Source: CAD feature listing. Evaluate the final solid. Frame: model axes, mm. Face numbers are marked on the shaded views. A direction names the side the tool comes from. Coordinates: 2 decimals unless noted, no trailing zeros. Write each loop counter-clockwise with the first axis right and the second up, starting at its lowest first coordinate (ties: lowest second). Pieces come first, ordered by that corner, then holes. Notation, with made-up numbers: M 51.5,-10.5 L 100.5,-10.5 A22 cw 100.5,17.5 Z; hole C -1,-37.5 d3. An arc over 180 degrees is marked long. Answer as CSV lines item,"result". Start each with the question number.
1. Line query: probe 1 along X at (y, z) = (211.5, 20.5); probe 2 along X at (y, z) = (152.5, -3); probe 3 along X at (y, z) = (285, -16). Output: solid intervals per line, ascending. Write a range as [from, to].
2. Mould query, pull axis X, two halves, no side actions, for the marked faces 3, 4, 5 and 6. Classes: pulls with the +X half, pulls with the -X half, needs draft (parallel to the pull), parting line crosses it, or undercut.
3. Section B-B on y = 429.5. Return the cut outline in (x, z), plus the area to 3 significant figures.
4. Section A-A on y = 214. Return the cut outline in (x, z).
5. Contact query for flat-ended pins moving along their axis: pin 1 Ø7 at (y, z) = (289.5, 11) entering from -X; pin 2 Ø5 at (x, y) = (40, 220) entering from -Z; pin 3 Ø11 at (y, z) = (262.5, 19.5) entering from +X. Output: stop coordinate, or through.
6. Section C-C on x = 36.5. Return the cut outline in (y, z), plus the area to 3 significant figures.
7. Reachability of the marked faces 1 and 2 from +Z, -Z, +X, -X, +Y, -Y: full face, straight path, thin tool, end or side. Return the list, or none.
Autodesk Inventor part; units mm, degrees
ref_plane "YZ Plane" through (0, 0, 0) normal (1, 0, 0) x (0, 1, 0)
ref_plane "XZ Plane" through (0, 0, 0) normal (0, 1, 0) x (-1, 0, 0)
ref_plane "XY Plane" through (0, 0, 0) normal (0, 0, 1) x (1, 0, 0)
sketch "草圖1" plane through (0, 0, 0) normal (0, 1, 0) x (-1, 0, 0)
  line L0 (-33.5, 27) -> (33.5, 27)
  line L1 (33.5, 27) -> (33.5, -27)
  line L2 (33.5, -27) -> (-33.5, -27)
  line L3 (-33.5, -27) -> (-33.5, 27)
  line L4 (-33.5, 27) -> (33.5, -27) construction
  line L5 (33.5, 27) -> (-33.5, -27) construction
  line L6 (43.5, -4.5) -> (33.5, -4.5)
  line L7 (33.5, -4.5) -> (33.5, 4.5)
  line L8 (33.5, 4.5) -> (43.5, 4.5)
  line L9 (43.5, 4.5) -> (43.5, -4.5)
  line L10 (-33.5, -4.5) -> (-43.5, -4.5)
  line L11 (-43.5, -4.5) -> (-43.5, 4.5)
  line L12 (-43.5, 4.5) -> (-33.5, 4.5)
  line L13 (-33.5, 4.5) -> (-33.5, -4.5)
  point P0 (0, 0)
  point P1 (33.5, 0)
  point P2 (-33.5, 0)
  point P3 (-33.5, 4.5)
  point P4 (-33.5, -4.5)
  dimension "d0" = 67
  dimension "d1" = 54
  dimension "d2" = 9
  dimension "d3" = 10
extrude "擠出1" add sketch "草圖1" along normal blind 450
sketch "草圖2" plane through (-33.5, 0, 27) normal (0, 0, 1) x (1, 0, 0)
  line L0 (0, 0) -> (0, 450)
  line L1 (0, 450) -> (67, 450)
  line L2 (67, 450) -> (67, 0)
  line L3 (67, 0) -> (0, 0)
  circle A0 centre (33.5, 222) radius 30
  line L4 (3.5, 222) -> (63.5, 222)
  line L5 (63.5, 222) -> (63.5, -38.0593)
  line L6 (63.5, -38.0593) -> (3.5, -38.0593)
  line L7 (3.5, -38.0593) -> (3.5, 222)
  point P0 (33.5, 0)
  point P1 (33.5, 0)
  dimension "d6" = 222
  dimension "d7" = 60
extrude "擠出2" cut sketch "草圖2" against normal through all contours L7 A0 L5 L3 | L3 L5 L6 L7 | L4 A0 | A0 L4
sketch "草圖3" plane through (-33.5, 450, 27) normal (0, 0, 1) x (1, 0, 0)
  line L0 (-67.0384, -320) -> (134.0384, -320)
  line L1 (134.0384, -320) -> (134.0384, -450)
  line L2 (134.0384, -450) -> (-67.0384, -450)
  line L3 (-67.0384, -450) -> (-67.0384, -320)
  point P0 (33.5, -450)
  point P1 (33.5, -450)
  dimension "d10" = 130
extrude "擠出3" cut sketch "草圖3" against normal through all
sketch "草圖4" plane through (33.5, 450, -27) normal (0, 0, -1) x (-1, 0, 0)
  circle A0 centre (33.5, -200) radius 30
  arc A1 (63.5, -228) -> (3.5, -228) centre (33.5, -228) ccw construction
  line L0 (63.5, -320) -> (3.5, -320)
  line L1 (3.5, -320) -> (3.5, -200)
  line L2 (3.5, -200) -> (63.5, -200)
  line L3 (63.5, -200) -> (63.5, -320)
  point P0 (33.5, -450)
  point P1 (63.5, -320)
  dimension "d13" = 28
  dimension "d14" = 60
sketch "草圖5" plane through (-33.5, 450, 27) normal (0, 0, 1) x (1, 0, 0)
  circle A0 centre (33.5, -198) radius 30
  arc A1 (63.5, -228) -> (3.5, -228) centre (33.5, -228) ccw construction
  line L0 (63.5, -320) -> (3.5, -320)
  line L1 (3.5, -320) -> (3.5, -198)
  line L2 (3.5, -198) -> (63.5, -198)
  line L3 (63.5, -198) -> (63.5, -320)
  point P0 (33.5, -450)
  point P1 (63.5, -320)
  dimension "d15" = 30
  dimension "d16" = 60
loft "斷面混成1" cut profiles "草圖4", "草圖5"
properties part number "Slider-8"
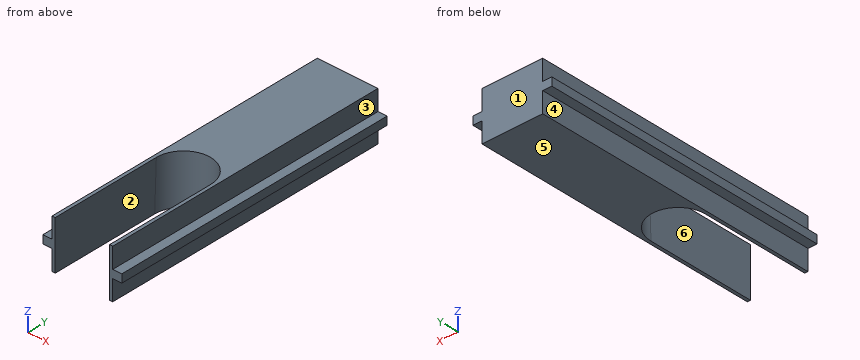
Values:
1,probe 1,"[-33.5, -30], [30, 33.5]"
1,probe 2,"[-43.5, -30], [30, 43.5]"
1,probe 3,"[-33.5, 33.5]"
2,face 3,"pulls with the +X half"
2,face 4,"pulls with the -X half"
2,face 5,"needs draft"
2,face 6,"undercut"
3,outline,"M -43.5,-4.5 L -33.5,-4.5 L -33.5,-27 L 33.5,-27 L 33.5,-4.5 L 43.5,-4.5 L 43.5,4.5 L 33.5,4.5 L 33.5,27 L -33.5,27 L -33.5,4.5 L -43.5,4.5 Z"
3,area,"3,800 mm²"
4,outline,"M -43.5,-4.5 L -33.5,-4.5 L -33.5,-27 L -30,-27 L -30,27 L -33.5,27 L -33.5,4.5 L -43.5,4.5 Z; M 30,-27 L 33.5,-27 L 33.5,-4.5 L 43.5,-4.5 L 43.5,4.5 L 33.5,4.5 L 33.5,27 L 30,27 Z"
5,pin 1,"x = -33.5"
5,pin 2,"z = -4.5"
5,pin 3,"x = 33.5"
6,outline,"M 130,-4.5 L 450,-4.5 L 450,4.5 L 130,4.5 Z"
6,area,"2,880 mm²"
7,face 1,"+Z, -Z, +X, -X, +Y"
7,face 2,"+Z, -Z, -Y"
